Source: CAD feature listing. Evaluate the final solid. Frame: model axes, mm. A direction names the side the tool comes from. Coordinates: 2 decimals unless noted, no trailing zeros. Order: outer loops, then holes, each group sorted by start corner. A loop starts at its lowest first (then second) coordinate and runs counter-clockwise, first axis right, second up. Notation, with made-up numbers: (-22.5, -11.5) - (1.5, -11.5) arc R16 cw to (1.5, -6.5) - close; hole circle Ø1 at (74, -27). An arc over 180 degrees is marked (long way). One line per question, with ' | ' between items. Start each with the question number.
(1) Line query: line 1 along Z through (x, y) = (0, 266); line 2 along X through (y, z) = (718, -5.5); line 3 along X through (y, z) = (750, -63.5). Output: solid intervals per line, ascending.
(2) Draft query along X for faces 4 (the cylindrical face through (55.06, 916.9, 247.96)), 5 (the flat face through (2, 0, 2)), 6 (the conical face through (20.23, 777.64, -154.06)). Return one class per face: +X half, -X half, draft (parallel to the pull), parting line (faces both ways), or undercut.
(3) Access query for faces 1 (the cylindrical face through (120.94, 828.4, 92.73)), 2 (the cylindrical face through (120.94, 383.68, 92.73)), 3 (the flat face through (2, 6.35, 2)). Directions: +Z, -Z, +X, -X, +Y, -Y. A direction counts if a zero-diameter tool reaches every point of the face in a straight line with its end or side. Return the directions, or none.
(4) Contact query for flat-ended pins moving along their axis: P1, Ø5, axis at y = 429, z = -32.5, coming from the -X side; P2, Ø6, axis at x = 57.5, y = 96, coming from the -Z side; P3, Ø2, axis at x = 16.5, y = 228, coming from the +Z side. Output: stop coordinate, or through.
(5) Section A-A (y = 737). Return the cut outline in (x, z).
Autodesk Inventor part; units mm, degrees
ref_plane "Work Plane1" through (-219.9994, 6.35, 0) normal (0, 0, 1) x (1, 0, 0)
ref_plane "YZ Plane" through (0, 0, 0) normal (1, 0, 0) x (0, 1, 0)
ref_plane "XZ Plane" through (0, 0, 0) normal (0, 1, 0) x (-1, 0, 0)
sketch "Sketch1" plane through (0, 0, 0) normal (0, 1, 0) x (-1, 0, 0)
  circle A0 centre (0, 0) radius 152.4
  circle A1 centre (0, 0) radius 146.05
  dimension "d0" = 304.8
  dimension "d1" = 6.35
extrude "Extrusion1" add sketch "Sketch1" along normal blind 863.6
extrude "Extrusion2" add sketch "Sketch1" along normal blind 6.35 contours A1
sketch "Sketch2" plane through (0, 6.35, 0) normal (0, 1, 0) x (1, 0, 0)
  line L0 (-219.9994, 0) -> (351.4578, 0)
  point P0 (0, 0)
ref_plane "Work Plane1" through (-219.9994, 6.35, 0) normal (0, 0, 1) x (1, 0, 0)
sketch "Sketch3" plane through (-219.9994, 6.35, 0) normal (0, 0, 1) x (1, 0, 0)
  line L0 (372.3994, 857.25) -> (67.5994, 857.25)
  line L1 (67.5994, 857.25) -> (67.5994, 913.13)
  line L2 (67.5994, 913.13) -> (-34.0006, 913.13)
  line L3 (-34.0006, 913.13) -> (-34.0006, 908.05)
  line L4 (-34.0006, 908.05) -> (67.5994, 857.25)
  line L5 (73.9494, 857.25) -> (366.0494, 857.25)
  line L6 (73.9494, 857.25) -> (-34.0006, 913.13)
  line L7 (219.9994, 947.7824) -> (219.9994, 874.9501)
  line L8 (372.3994, 857.25) -> (67.5994, 857.25)
  line L9 (372.3994, -6.35) -> (67.5994, -6.35)
  line L10 (67.5994, -6.35) -> (67.5994, 857.25)
  line L11 (67.5994, -6.35) -> (67.5994, 857.25)
  line L12 (67.5994, 771.9109) -> (19.9744, 762)
  line L13 (19.9744, 762) -> (16.7994, 777.2569)
  line L14 (16.7994, 777.2569) -> (67.5994, 787.8285)
  line L15 (67.5994, -6.35) -> (67.5994, 857.25)
  point P0 (219.9994, -6.35)
  point P1 (67.5994, 787.8285)
  dimension "d6" = 55.88
  dimension "d7" = 101.6
  dimension "d8" = 5.08
revolve "Revolution1" add sketch "Sketch3" angle 360 about axis through (0, 954.1324, 0) along (0, -1, 0) contours L10 L12 L13 L14 | L0 L1 L6 | L4 L3 L6 L1
properties part number "Trash bin casing X1" material "Stainless Steel"
Response values:
1) line 1: z = -152.4 to -146.05, 146.05 to 152.4 | line 2: x = -152.3 to -145.95, 145.95 to 152.3 | line 3: x = -138.54 to -131.52, 131.52 to 138.54
2) face 4: parting line | face 5: draft | face 6: undercut
3) face 1: none | face 2: -Y | face 3: +Y
4) P1: stops at x = -149.42 | P2: stops at z = -142.32 | P3: stops at z = 151.61
5) outline: circle Ø304.8 at (0, 0); hole circle Ø292.1 at (0, 0)
